Here's how the part is built. I have some questions about the finished solid (model axes, mm). A direction names the side the tool comes from. Round coordinates to 2 decimals unless told otherwise and drop trailing zeros. Loops run counter-clockwise (first coordinate to the right, second up) from the corner with the lowest first, then second, coordinate; pieces in that order, holes last. Notation, with made-up numbers: M -6.5,-26 L 24.5,-26 A23 cw 24.5,10 Z; hole C 63,37.25 d8. An arc over 180 degrees is marked long. Use a Markdown table: item, result.
```python
from build123d import *

# Parameters (mm, degrees)
SKETCH1_W           = 35
SKETCH1_H           = 35
SKETCH1_W_2         = 31.4
SKETCH1_H_2         = 31.4
BOSS_EXTRUDE1_DEPTH = 380
SKETCH3_R           = 2
CUT_EXTRUDE1_DEPTH  = 383.009489411
SKETCH4_R           = 2
CUT_EXTRUDE2_DEPTH  = 383.009489411
SKETCH13_R          = 15
CUT_EXTRUDE10_DEPTH = 383.009489411
SKETCH14_R          = 2.25
CUT_EXTRUDE11_DEPTH = 383.009489411
LPATTERN1_COUNT     = 6
LPATTERN1_PITCH     = 45
SKETCH16_R          = 2.25
CUT_EXTRUDE13_DEPTH = 383.009489411
SKETCH17_R          = 15
CUT_EXTRUDE14_DEPTH = 383.009489411
LPATTERN2_COUNT     = 7
LPATTERN2_PITCH     = 45
BOSS_EXTRUDE2_START = -1.8
SKETCH18_R          = 15
BOSS_EXTRUDE2_DEPTH = 1.8
SKETCH19_R          = 4
CUT_EXTRUDE15_DEPTH = 382.848778969
CUT_EXTRUDE16_REACH = 384.009
SKETCH20_R          = 1
SKETCH20_R_2        = 1.25


with BuildPart() as part:
    # Sketch1 → Boss-Extrude1 (new body)
    with BuildSketch(Plane(origin=(0, 0, 0), x_dir=(1, 0, 0), z_dir=(0, 1, 0))):
        Rectangle(SKETCH1_W, SKETCH1_H)
        Rectangle(SKETCH1_W_2, SKETCH1_H_2, mode=Mode.SUBTRACT)
    extrude(amount=BOSS_EXTRUDE1_DEPTH)

    # Sketch3 → Cut-Extrude1 (cut, through all)
    with BuildSketch(Plane.XY.offset(17.5)):
        with Locations((0, 10)):
            Circle(SKETCH3_R)
    extrude(amount=-CUT_EXTRUDE1_DEPTH, mode=Mode.SUBTRACT)

    # Sketch4 → Cut-Extrude2 (cut, through all)
    with BuildSketch(Plane(origin=(17.5, 0, 0), x_dir=(0, 0, -1), z_dir=(1, 0, 0))):
        with Locations((0, 10)):
            Circle(SKETCH4_R)
    extrude(amount=-CUT_EXTRUDE2_DEPTH, mode=Mode.SUBTRACT)

    # Sketch13 → Cut-Extrude10 (cut, through all)
    with BuildSketch(Plane.ZY.offset(17.5)):
        with Locations((0, 95.5)):
            Circle(SKETCH13_R)
    cut_extrude10 = extrude(amount=-CUT_EXTRUDE10_DEPTH, mode=Mode.SUBTRACT)

    # Sketch14 → Cut-Extrude11 (cut, through all)
    with BuildSketch(Plane(origin=(17.5, 0, 0), x_dir=(0, 0, -1), z_dir=(1, 0, 0))):
        with Locations((0, 372)):
            Circle(SKETCH14_R)
        with Locations((0, 356)):
            Circle(SKETCH14_R)
        with Locations((0, 46)):
            Circle(SKETCH14_R)
        with Locations((0, 30)):
            Circle(SKETCH14_R)
    extrude(amount=-CUT_EXTRUDE11_DEPTH, mode=Mode.SUBTRACT)

    # LPattern1: Cut-Extrude10 ×6
    with Locations(*[(0, i * LPATTERN1_PITCH, 0) for i in range(1, LPATTERN1_COUNT)]):
        add(cut_extrude10, mode=Mode.SUBTRACT)

    # Sketch16 → Cut-Extrude13 (cut, through all)
    with BuildSketch(Plane.XY.offset(17.5)):
        with Locations((0, 46)):
            Circle(SKETCH16_R)
        with Locations((0, 30)):
            Circle(SKETCH16_R)
    extrude(amount=-CUT_EXTRUDE13_DEPTH, mode=Mode.SUBTRACT)

    # Sketch17 → Cut-Extrude14 (cut, through all)
    with BuildSketch(Plane.XY.offset(17.5)):
        with Locations((0, 73)):
            Circle(SKETCH17_R)
    cut_extrude14 = extrude(amount=-CUT_EXTRUDE14_DEPTH, mode=Mode.SUBTRACT)

    # LPattern2: Cut-Extrude14 ×7
    with Locations(*[(0, i * LPATTERN2_PITCH, 0) for i in range(1, LPATTERN2_COUNT)]):
        add(cut_extrude14, mode=Mode.SUBTRACT)

    # Sketch18 → Boss-Extrude2 (add)
    with BuildSketch(Plane(origin=(0, 0, -17.5), x_dir=(-1, 0, 0), z_dir=(0, 0, -1)).offset(BOSS_EXTRUDE2_START)):
        with Locations(Location((0, 163, 0), (0, 0, 180))):
            Circle(SKETCH18_R)
    extrude(amount=BOSS_EXTRUDE2_DEPTH)

    # Sketch19 → Cut-Extrude15 (cut, through all)
    with BuildSketch(Plane.XY.offset(-15.7)):
        with Locations((0, 163)):
            Circle(SKETCH19_R)
    extrude(amount=-CUT_EXTRUDE15_DEPTH, mode=Mode.SUBTRACT)

    # Sketch20 → Cut-Extrude16 (cut, up to next)
    with BuildSketch(Plane(origin=(0, 0, -17.5), x_dir=(-1, 0, 0), z_dir=(0, 0, -1)), mode=Mode.PRIVATE) as cut_extrude16_sk1:
        with Locations((0, 171)):
            Circle(SKETCH20_R)
    cut_extrude16_tool1 = extrude(cut_extrude16_sk1.sketch, amount=-CUT_EXTRUDE16_REACH, mode=Mode.PRIVATE) & part.part
    # Sketch20 → Cut-Extrude16 (cut, up to next)
    with BuildSketch(Plane(origin=(0, 0, -17.5), x_dir=(-1, 0, 0), z_dir=(0, 0, -1)), mode=Mode.PRIVATE) as cut_extrude16_sk2:
        with Locations((0, 155)):
            Circle(SKETCH20_R)
    cut_extrude16_tool2 = extrude(cut_extrude16_sk2.sketch, amount=-CUT_EXTRUDE16_REACH, mode=Mode.PRIVATE) & part.part
    # Sketch20 → Cut-Extrude16 (cut, up to next)
    with BuildSketch(Plane(origin=(0, 0, -17.5), x_dir=(-1, 0, 0), z_dir=(0, 0, -1)), mode=Mode.PRIVATE) as cut_extrude16_sk3:
        with Locations((8, 163)):
            Circle(SKETCH20_R)
    cut_extrude16_tool3 = extrude(cut_extrude16_sk3.sketch, amount=-CUT_EXTRUDE16_REACH, mode=Mode.PRIVATE) & part.part
    # Sketch20 → Cut-Extrude16 (cut, up to next)
    with BuildSketch(Plane(origin=(0, 0, -17.5), x_dir=(-1, 0, 0), z_dir=(0, 0, -1)), mode=Mode.PRIVATE) as cut_extrude16_sk4:
        with Locations((-8, 163)):
            Circle(SKETCH20_R)
    cut_extrude16_tool4 = extrude(cut_extrude16_sk4.sketch, amount=-CUT_EXTRUDE16_REACH, mode=Mode.PRIVATE) & part.part
    # Sketch20 → Cut-Extrude16 (cut, up to next)
    with BuildSketch(Plane(origin=(0, 0, -17.5), x_dir=(-1, 0, 0), z_dir=(0, 0, -1)), mode=Mode.PRIVATE) as cut_extrude16_sk5:
        with Locations((-7.778174593, 155.221825407)):
            Circle(SKETCH20_R_2)
    cut_extrude16_tool5 = extrude(cut_extrude16_sk5.sketch, amount=-CUT_EXTRUDE16_REACH, mode=Mode.PRIVATE) & part.part
    # Sketch20 → Cut-Extrude16 (cut, up to next)
    with BuildSketch(Plane(origin=(0, 0, -17.5), x_dir=(-1, 0, 0), z_dir=(0, 0, -1)), mode=Mode.PRIVATE) as cut_extrude16_sk6:
        with Locations((7.778174593, 155.221825407)):
            Circle(SKETCH20_R_2)
    cut_extrude16_tool6 = extrude(cut_extrude16_sk6.sketch, amount=-CUT_EXTRUDE16_REACH, mode=Mode.PRIVATE) & part.part
    # Sketch20 → Cut-Extrude16 (cut, up to next)
    with BuildSketch(Plane(origin=(0, 0, -17.5), x_dir=(-1, 0, 0), z_dir=(0, 0, -1)), mode=Mode.PRIVATE) as cut_extrude16_sk7:
        with Locations((7.778174593, 170.778174593)):
            Circle(SKETCH20_R_2)
    cut_extrude16_tool7 = extrude(cut_extrude16_sk7.sketch, amount=-CUT_EXTRUDE16_REACH, mode=Mode.PRIVATE) & part.part
    # Sketch20 → Cut-Extrude16 (cut, up to next)
    with BuildSketch(Plane(origin=(0, 0, -17.5), x_dir=(-1, 0, 0), z_dir=(0, 0, -1)), mode=Mode.PRIVATE) as cut_extrude16_sk8:
        with Locations((-7.778174593, 170.778174593)):
            Circle(SKETCH20_R_2)
    cut_extrude16_tool8 = extrude(cut_extrude16_sk8.sketch, amount=-CUT_EXTRUDE16_REACH, mode=Mode.PRIVATE) & part.part
    add(cut_extrude16_tool1.solids().sort_by_distance((0, 171, -17.5))[0], mode=Mode.SUBTRACT)
    add(cut_extrude16_tool2.solids().sort_by_distance((0, 155, -17.5))[0], mode=Mode.SUBTRACT)
    add(cut_extrude16_tool3.solids().sort_by_distance((-8, 163, -17.5))[0], mode=Mode.SUBTRACT)
    add(cut_extrude16_tool4.solids().sort_by_distance((8, 163, -17.5))[0], mode=Mode.SUBTRACT)
    add(cut_extrude16_tool5.solids().sort_by_distance((7.778175, 155.221825, -17.5))[0], mode=Mode.SUBTRACT)
    add(cut_extrude16_tool6.solids().sort_by_distance((-7.778175, 155.221825, -17.5))[0], mode=Mode.SUBTRACT)
    add(cut_extrude16_tool7.solids().sort_by_distance((-7.778175, 170.778175, -17.5))[0], mode=Mode.SUBTRACT)
    add(cut_extrude16_tool8.solids().sort_by_distance((7.778175, 170.778175, -17.5))[0], mode=Mode.SUBTRACT)


solid = part.part
```
Q1. For faces 4 (the cylindrical face through (-16.613, 170.857, -3.252)), 5 (the flat face through (-15.7, 103, 14)), which set-ups out of +Z, -Z, +X, -X, +Y, -Y let a thin tool reach every point of the face, with its end or its side?
Return value:
| item | result |
|---|---|
| face 4 | +X, -X |
| face 5 | +Y, -Y |
Q2. Imagine slicing it at A-A, the plane y = 208. Please give me the cut outline in (x, z).
Return value:
| item | result |
|---|---|
| outline | M -17.5,-17.5 L -15,-17.5 L -15,-15.7 L -15.7,-15.7 L -15.7,15.7 L -15,15.7 L -15,17.5 L -17.5,17.5 Z; M 15,-17.5 L 17.5,-17.5 L 17.5,17.5 L 15,17.5 L 15,15.7 L 15.7,15.7 L 15.7,-15.7 L 15,-15.7 Z |
Q3. Will this pin go through, and if not, where does the flat tip stop? P1, Ø18, axis at y = 275.5, z = 0, coming from the +X side.
Return value:
| item | result |
|---|---|
| P1 | passes through |
Q4. We'd pull the mould along Z, two halves only. Please class faces 1 (the cylindrical face through (16.587, 215.857, -3.252)), 2 (the flat face through (0, 187, -17.5)), 3 (the cylindrical face through (-1.953, 357.872, -16.587)): pulls with the +Z half, pulls with the -Z half, needs draft (parallel to the pull), parting line crosses it, or undercut.
Return value:
| item | result |
|---|---|
| face 1 | undercut |
| face 2 | pulls with the -Z half |
| face 3 | needs draft |
Q5. I need wall thicknesses on line 1 (Z direction, x = -8.5, y = 282); line 2 (Z direction, x = -17, y = 356). Which ranges of each line are inside material? Lowest first, please. Write a range as from..to.
Return value:
| item | result |
|---|---|
| line 1 | z = -17.5..-15.7, 15.7..17.5 |
| line 2 | z = -17.5..-2.25, 2.25..17.5 |
Q6. Imagine slicing it at B-B, the plane z = 5.5. Give the number of separate pieces and of enclosed holes in the cut face, then the cut area to 3 significant figures.
Return value:
| item | result |
|---|---|
| separate pieces | 14 |
| enclosed holes | 0 |
| area | 765 mm^2 |
